from build123d import *

# Parameters (mm, degrees)
SKETCH_1_W                         = 400
SKETCH_1_H                         = 142
SM_BASE_FLANGE_1_DEPTH             = 0.7
SM_EDGE_FLANGE_1_STRIP_W           = 3.2
SM_EDGE_FLANGE_1_STRIP_H           = 0.7
SM_EDGE_FLANGE_1_STRIP_CUT_DEPTH   = 400
SM_EDGE_FLANGE_1_STRIP_2_W         = 3.2
SM_EDGE_FLANGE_1_STRIP_2_H         = 0.7
SM_EDGE_FLANGE_1_STRIP_CUT_2_DEPTH = 400
SM_EDGE_FLANGE_1_DEPTH             = 400
SM_EDGE_FLANGE_1_BEND_DEPTH        = 400
SKETCH_17_R                        = 3
CUT_EXTRUDE_1_DEPTH                = 10
CUT_EXTRUDE_START                  = -10
SKETCH_18_R                        = 3
CUT_EXTRUDE_2_DEPTH                = 10
SKETCH_19_R                        = 30
SKETCH_19_R_2                      = 2
CUT_EXTRUDE_4_DEPTH                = 10


# Sheet-metal steps are written as plain solids
with BuildPart() as part:
    # 草图1 → 基体-法兰1 (new body)
    with BuildSketch(Plane(origin=(0, 0, 0), x_dir=(1, 0, 0), z_dir=(0, 1, 0))):
        Rectangle(SKETCH_1_W, SKETCH_1_H)
    extrude(amount=-SM_BASE_FLANGE_1_DEPTH)

    # 边线-法兰1 strip (across the edge) → 边线-法兰1 strip cut (cut)
    with BuildSketch(Plane(origin=(200, 0, -71), x_dir=(0, 0, 1), z_dir=(-1, 0, 0))):
        with Locations((-0.7, -0.35)):
            Rectangle(SM_EDGE_FLANGE_1_STRIP_W, SM_EDGE_FLANGE_1_STRIP_H)
    extrude(amount=SM_EDGE_FLANGE_1_STRIP_CUT_DEPTH, mode=Mode.SUBTRACT)

    # 边线-法兰1 strip 2 (across the edge) → 边线-法兰1 strip cut 2 (cut)
    with BuildSketch(Plane(origin=(-200, 0, 71), x_dir=(0, 0, -1), z_dir=(1, 0, 0))):
        with Locations((-0.7, -0.35)):
            Rectangle(SM_EDGE_FLANGE_1_STRIP_2_W, SM_EDGE_FLANGE_1_STRIP_2_H)
    extrude(amount=SM_EDGE_FLANGE_1_STRIP_CUT_2_DEPTH, mode=Mode.SUBTRACT)

    # 边线-法兰1 section (across the edge) → 边线-法兰1 (add)
    with BuildSketch(Plane(origin=(200, 0, -71), x_dir=(0, 0, 1), z_dir=(-1, 0, 0))):
        with BuildLine():
            Line((0, 0.2), (0, 14.3))
            Line((0, 14.3), (0.7, 14.3))
            Line((0.7, 14.3), (0.7, 0.2))
            ThreePointArc((0.7, 0.2), (0.758578644, 0.058578644), (0.9, 0))
            Line((0.9, 0), (0.9, -0.7))
            ThreePointArc((0.9, -0.7), (0.263603897, -0.436396103), (0, 0.2))
        make_face()
    extrude(amount=SM_EDGE_FLANGE_1_DEPTH)

    # 边线-法兰1 section 2 (across the edge) → 边线-法兰1 bend (add)
    with BuildSketch(Plane(origin=(-200, 0, 71), x_dir=(0, 0, -1), z_dir=(1, 0, 0))):
        with BuildLine():
            Line((0, 0.2), (0, 14.3))
            Line((0, 14.3), (0.7, 14.3))
            Line((0.7, 14.3), (0.7, 0.2))
            ThreePointArc((0.7, 0.2), (0.758578644, 0.058578644), (0.9, 0))
            Line((0.9, 0), (0.9, -0.7))
            ThreePointArc((0.9, -0.7), (0.263603897, -0.436396103), (0, 0.2))
        make_face()
    extrude(amount=SM_EDGE_FLANGE_1_BEND_DEPTH)

    # 草图17 → 切除-拉伸1 (cut)
    with BuildSketch(Plane(origin=(0, 0, -71), x_dir=(-1, 0, 0), z_dir=(0, 0, -1))):
        with Locations(Location((-194.5, 8.8, 0), (0, 0, 90))):
            Circle(SKETCH_17_R)
        with Locations(Location((0, 8.8, 0), (0, 0, 90))):
            Circle(SKETCH_17_R)
        with Locations(Location((194.5, 8.8, 0), (0, 0, 270))):
            Circle(SKETCH_17_R)
    extrude(amount=-CUT_EXTRUDE_1_DEPTH, mode=Mode.SUBTRACT)

    # 草图18 → 切除-拉伸2 (cut)
    with BuildSketch(Plane.XY.offset(71).offset(CUT_EXTRUDE_START)):
        with Locations(Location((-194.5, 8.8, 0), (0, 0, 270))):
            Circle(SKETCH_18_R)
        with Locations(Location((0, 8.8, 0), (0, 0, 90))):
            Circle(SKETCH_18_R)
        with Locations(Location((194.5, 8.8, 0), (0, 0, 90))):
            Circle(SKETCH_18_R)
    extrude(amount=CUT_EXTRUDE_2_DEPTH, mode=Mode.SUBTRACT)

    # 草图19 → 切除-拉伸4 (cut)
    with BuildSketch(Plane.XZ.offset(0.7)):
        with Locations(Location((145, 0, 0), (0, 0, 270))):
            Circle(SKETCH_19_R)
        with Locations(Location((127.5, 30.310889132, 0), (0, 0, 270))):
            Circle(SKETCH_19_R_2)
        with Locations(Location((180, 0, 0), (0, 0, 270))):
            Circle(SKETCH_19_R_2)
        with Locations(Location((127.5, -30.310889132, 0), (0, 0, 270))):
            Circle(SKETCH_19_R_2)
    extrude(amount=-CUT_EXTRUDE_4_DEPTH, mode=Mode.SUBTRACT)


solid = part.part
The model under review builds one solid part; all positions refer to its coordinate system, in mm. A direction names the side the tool comes from. Coordinates: 2 decimals unless noted, no trailing zeros. Loops run counter-clockwise (first coordinate to the right, second up) from the corner with the lowest first, then second, coordinate; pieces in that order, holes last. Notation, with made-up numbers: (-8, 31) -> (3, 31) arc R18 ccw to (3, 57) -> close; hole circle Ø11 at (-12, 85). An arc over 180 degrees is marked (long way). Use a Markdown table: item, result. Add a question column.
1. To check wall thickness, follow line 1 (X direction, y = 8.8, z = -70.75); line 2 (X direction, y = -0.45, z = 0); line 3 (Z direction, x = 139, y = 4.5). State the ranges of each line that lie inside material, in increasing order.
2. Draft analysis for pull direction Z (two halves, no side actions). For faces 3 (the face through (200, -0.4, -0.3)), 4 (the face through (-3, 7, 71)), 5 (the face through (-3, 0, -1)), state which applies: pulls with the +Z half, pulls with the -Z half, needs draft (parallel to the pull), parting line crosses it, or undercut.
3. Clearance check with flat-ended pins moving along their axes: pin 1 Ø2.5 at (x, z) = (127.5, 30.31) entering from +Y; pin 2 Ø5 at (x, z) = (180, 0) entering from +Y. State where each tip first meets the part, or that it passes through.
4. Machinability: for faces 1 (the face through (-3, 7, 70.3)), 2 (the face through (3, 7, -71)), which of the approach directions +Z, -Z, +X, -X, +Y, -Y give a long, thin tool a straight path to every point of the face, cutting with its end or side? Answer none if there is none.
5. Add section C-C on x = 53. Write out the cut boundary in (y, z), plus the area to 3 significant figures.
6. Add section D-D on z = 61. Write out the cut boundary in (x, y), plus the area to 3 significant figures.
7. Add section B-B on x = 145. Write out the cut boundary in (y, z).
8. Add section A-A on y = 8.8. Give the number of separate pieces and of enclosed holes in the cut face, plus the area to 3 significant figures.
Returned:
| question | item | result |
|---|---|---|
| 1 | line 1 | x = -200 to -197.5, -191.5 to -3, 3 to 191.5, 197.5 to 200 |
| 1 | line 2 | x = -200 to 115, 175 to 178, 182 to 200 |
| 1 | line 3 | z = -71 to -70.3, 70.3 to 71 |
| 2 | face 3 | needs draft |
| 2 | face 4 | pulls with the +Z half |
| 2 | face 5 | undercut |
| 3 | pin 1 | passes through |
| 3 | pin 2 | stops at y = 0 |
| 4 | face 1 | +X, -X, +Y |
| 4 | face 2 | -Z, +X, -X, +Y, -Y |
| 5 | outline | (-0.7, -70.1) arc R0.9 ccw to (0.2, -71) -> (14.3, -71) -> (14.3, -70.3) -> (0.2, -70.3) arc R0.2 cw to (0, -70.1) -> (0, 70.1) arc R0.2 cw to (0.2, 70.3) -> (14.3, 70.3) -> (14.3, 71) -> (0.2, 71) arc R0.9 ccw to (-0.7, 70.1) -> close |
| 5 | area | 119 mm² |
| 6 | outline | (-200, -0.7) -> (200, -0.7) -> (200, 0) -> (-200, 0) -> close |
| 6 | area | 280 mm² |
| 7 | outline | (-0.7, -70.1) arc R0.9 ccw to (0.2, -71) -> (14.3, -71) -> (14.3, -70.3) -> (0.2, -70.3) arc R0.2 cw to (0, -70.1) -> (0, -30) -> (-0.7, -30) -> close; (-0.7, 30) -> (0, 30) -> (0, 70.1) arc R0.2 cw to (0.2, 70.3) -> (14.3, 70.3) -> (14.3, 71) -> (0.2, 71) arc R0.9 ccw to (-0.7, 70.1) -> close |
| 8 | separate pieces | 8 |
| 8 | enclosed holes | 0 |
| 8 | area | 535 mm² |
